Autodesk Inventor part; units mm, degrees
ref_plane "YZ Plane" through (0, 0, 0) normal (1, 0, 0) x (0, 1, 0)
ref_plane "XZ Plane" through (0, 0, 0) normal (0, 1, 0) x (-1, 0, 0)
ref_plane "XY Plane" through (0, 0, 0) normal (0, 0, 1) x (1, 0, 0)
sketch "Sketch1" plane through (0, 0, 0) normal (0, 0, 1) x (1, 0, 0)
  circle A0 centre (0, 0) radius 6.35
  arc A1 (0, 9.525) -> (0, -9.525) centre (0, 0) ccw
  line L0 (0, -9.525) -> (19.05, -9.525)
  line L1 (19.05, -9.525) -> (19.05, 9.525)
  line L2 (19.05, 9.525) -> (0, 9.525)
  dimension "d0" = 12.7
  dimension "d1" = 19.05
  dimension "d2" = 19.05
  dimension "d3" = 19.05
extrude "Extrusion1" add sketch "Sketch1" along normal blind 9.525
fillet "Fillet1" radius 6.35 1 edges at (19.05, -9.525, 4.7625)
sketch "Sketch2" plane through (0, 9.525, 0) normal (0, 1, 0) x (1, 0, 0)
  line L0 (0, 0) -> (19.05, 0)
  line L1 (0, 0) -> (0, -9.525)
  line L2 (19.05, -9.525) -> (0, -9.525)
  line L3 (19.05, 0) -> (19.05, -9.525)
  line L4 (6.35, 0) -> (6.35, -9.525)
  point P0 (0, 0)
  point P1 (14.2875, -4.7625)
  dimension "d7" = 4.7625
  dimension "d9" = 9.525
  dimension "d17" = 7.9375
hole "Hole1" at (14.2875, 9.525, 4.7625) direction (0, -1, 0) diameter 4.9784 depth 11.1125 tip angle 118
mirror "Mirror1" about plane through (0, 0, 0) normal (1, 0, 0) of "Extrusion1", "Hole1", "Fillet1"
properties part number "WheelSuspensionHub" material "Aluminum 6061"
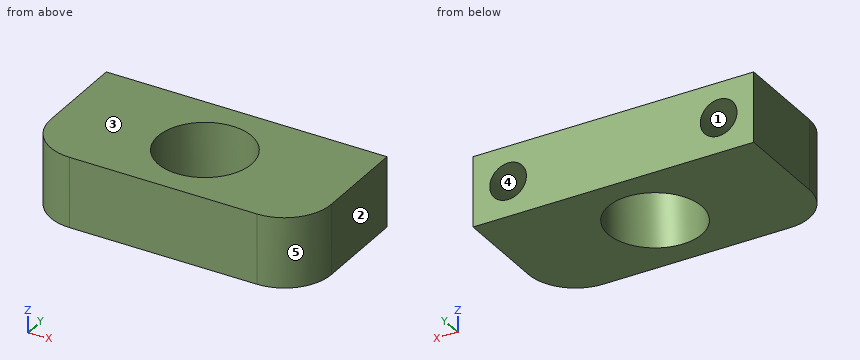
Source: CAD feature listing. Evaluate the final solid. Frame: model axes, mm. Face numbers are marked on the shaded views. A direction names the side the tool comes from. Coordinates: 2 decimals unless noted, no trailing zeros. Loops run counter-clockwise (first coordinate to the right, second up) from the corner with the lowest first, then second, coordinate; pieces in that order, holes last. Notation, with made-up numbers: M 83.25,-25 L 89.25,-25 A28 ccw 89.25,10 Z; hole C 25.25,88 d5. An arc over 180 degrees is marked long. Use CSV: the item, a comma, the result in double quotes.
(1) Line query: line 1 (Y direction, x = 0, z = 7.5) (3 decimals); line 2 (X direction, y = 0, z = 3); line 3 (Y direction, x = -2, z = 3.25) (3 decimals). Output: solid intervals per line, ascending. Write a range as [from, to].
Answers follow:
line 1,"[-9.525, -6.35], [6.35, 9.525]"
line 2,"[-19.05, -16.05], [-12.53, -6.35], [6.35, 12.53], [16.05, 19.05]"
line 3,"[-9.525, -6.027], [6.027, 9.525]"
(2) Cut plane B-B on z = 1.25. Return loops of the section in (x, y) (3 decimals).
Answers follow:
outline,"M -19.05,-3.175 A6.35 ccw -12.7,-9.525 L 12.7,-9.525 A6.35 ccw 19.05,-3.175 L 19.05,9.525 L -19.05,9.525 Z; hole C 0,0 d12.7"
(3) Draft query along X for the marked faces 1, 2 and 3. Return one class per face: pulls with the +X half, pulls with the -X half, needs draft (parallel to the pull), parting line crosses it, or undercut.
Answers follow:
face 1,"undercut"
face 2,"pulls with the +X half"
face 3,"needs draft"
(4) Reachability of the marked faces 4 and 5 from +Z, -Z, +X, -X, +Y, -Y: full face, straight path, thin tool, end or side. Return the list, or none.
Answers follow:
face 4,"+Y"
face 5,"+Z, -Z, +X, -Y"
(5) Cut plane C-C on x = -5. Return loops of the section in (y, z) (3 decimals).
Answers follow:
outline,"M -9.525,0 L -3.914,0 L -3.914,9.525 L -9.525,9.525 Z; M 3.914,0 L 9.525,0 L 9.525,9.525 L 3.914,9.525 Z"
(6) Cut plane A-A on y = 1. Give the number of separate pieces and of enclosed holes in the cut face, and give its area (3 significant figures).
Answers follow:
separate pieces,"2"
enclosed holes,"2"
area,"205 mm²"
(7) Cut plane D-D on y = -5.25. Return loops of the section in (x, z) (3 decimals), and give its area (3 significant figures).
Answers follow:
outline,"M -18.701,0 L -3.572,0 L -3.572,9.525 L -18.701,9.525 Z; M 3.572,0 L 18.701,0 L 18.701,9.525 L 3.572,9.525 Z"
area,"288 mm²"
